from build123d import *

# Parameters (mm, degrees)
BOSS_EXTRUDE1_DEPTH           = 10
FILLET1_R                     = 5
CHAMFER1_SIZE                 = 1.5
CSK_FOR_M4_SFHCS1_D           = 4.8
CSK_FOR_M4_SFHCS1_CSINK_D     = 8.96
CSK_FOR_M4_SFHCS1_CSINK_ANGLE = 90
CSK_FOR_M4_SFHCS2_D           = 4.8
CSK_FOR_M4_SFHCS2_DEPTH       = 9.6
CSK_FOR_M4_SFHCS2_CSINK_D     = 8.96
CSK_FOR_M4_SFHCS2_CSINK_ANGLE = 90


with BuildPart() as part:
    # Sketch1 → Boss-Extrude1 (new body)
    with BuildSketch(Plane(origin=(0, 0, 0), x_dir=(1, 0, 0), z_dir=(0, 1, 0))):
        Polygon((-30, -17.5), (-30, -27.5), (30, -27.5), (30, -17.5), (20, -17.5), (20, 27.5), (10.4, 27.5), (10.4, 7.1), (-10.4, 7.1), (-10.4, 27.5), (-20, 27.5), (-20, -17.5), align=None)
    extrude(amount=BOSS_EXTRUDE1_DEPTH)

    # Fillet1
    fillet1_edges = [part.edges().sort_by_distance(p)[0] for p in [
        (-15.2, 0, -27.5),
        (15.2, 0, -27.5),
        (-15.2, 10, -27.5),
        (15.2, 10, -27.5),
        (0, 10, -7.1),
        (0, 0, -7.1),
    ]]
    fillet(fillet1_edges, radius=FILLET1_R - 0.0001)  # a hair under: the kernel refuses the full size

    # Chamfer1
    chamfer1_edges = [part.edges().sort_by_distance(p)[0] for p in [
        (30, 0, 22.5),
        (-30, 0, 22.5),
        (-30, 10, 22.5),
        (30, 10, 22.5),
    ]]
    chamfer(chamfer1_edges, length=CHAMFER1_SIZE)

    # CSK for M4 SFHCS1 (through all)
    with Locations(Plane(origin=(0, 0, 17.5), x_dir=(-1, 0, 0), z_dir=(0, 0, -1))):
        with Locations((-25, 5), (25, 5)):
            CounterSinkHole(CSK_FOR_M4_SFHCS1_D / 2, CSK_FOR_M4_SFHCS1_CSINK_D / 2, counter_sink_angle=CSK_FOR_M4_SFHCS1_CSINK_ANGLE)

    # CSK for M4 SFHCS2
    with Locations(Plane.ZY.offset(20)):
        with Locations((-22.5, 5)):
            csk_for_m4_sfhcs2 = CounterSinkHole(CSK_FOR_M4_SFHCS2_D / 2, CSK_FOR_M4_SFHCS2_CSINK_D / 2, depth=CSK_FOR_M4_SFHCS2_DEPTH, counter_sink_angle=CSK_FOR_M4_SFHCS2_CSINK_ANGLE)

    # Mirror1: CSK for M4 SFHCS2 across plane
    add(csk_for_m4_sfhcs2.mirror(Plane(origin=(0, 0, 0), x_dir=(0, 0, 1), z_dir=(1, 0, 0))), mode=Mode.SUBTRACT)


solid = part.part
Geometry check sheet. Reference: the model listing, model coordinates, mm. A direction names the side the tool comes from. Give positions to 0.01 mm unless a question says otherwise; leave off trailing zeros. Write each loop counter-clockwise with the first axis right and the second up, starting at its lowest first coordinate (ties: lowest second). Pieces come first, ordered by that corner, then holes. Notation, with made-up numbers: M 32.5,49 L 84.5,49 A22 ccw 84.5,55 Z; hole C -14,69 d5. An arc over 180 degrees is marked long. Answer as CSV lines item,"result". Start each with the question number.
Q1. Section check A-A, the plane x = 25. Record the cut outline in (y, z).
Q2. Section check B-B, the plane z = 22. Record the cut outline in (x, y), then the cut area to 3 significant figures.
Q3. Go/stop test with flat-tipped pins: pin 1 (5 mm diameter, centred on x = 25.5, y = 3, fed in from -Z); pin 2 (3 mm diameter, centred on x = -26, y = 6.5, fed in from -Z); pin 3 (5 mm diameter, centred on y = 1, z = 3.5, fed in from +X). Record where each tip stops, or that it passes through.
Q4. Tool access check on faces 1 (the face through (-20.5, 3.8, 17.5)), 2 (the face through (-0.15, 8.5, -5.67)), 3 (the face through (0, 0, 8)), 4 (the face through (23.959, 0.486, 17.5)). Record the directions out of +Z, -Z, +X, -X, +Y, -Y that give a thin tool (end or side, any length) a straight path to the whole face; none if there is none.
Q5. Material ranges on L1, parallel to X at y = 5, z = 24; L2, parallel to X at y = 9.75, z = -8.5; L3, parallel to Y at x = 16.5, z = -22.5, recorded low to high.
Q6. Release check for a two-part mould opening along Y. For faces 5 (the face through (-15.27, 8.5, -26.07)), 6 (the face through (14.11, 5.72, -24.79)), 7 (the face through (-20, 5, 0)) record: pulls with the +Y half, pulls with the -Y half, needs draft (parallel to the pull), parting line crosses it, or undercut.
Geometry says:
1,outline,"M 0,17.5 L 0.52,17.5 L 2.6,19.58 L 2.6,27.5 L 0,27.5 Z; M 7.4,19.58 L 9.48,17.5 L 10,17.5 L 10,27.5 L 7.4,27.5 Z"
2,outline,"M -30,1.5 L -28.5,0 L 28.5,0 L 30,1.5 L 30,8.5 L 28.5,10 L -28.5,10 L -30,8.5 Z; hole C -25,5 d4.8; hole C 25,5 d4.8"
2,area,"559 mm^2"
3,pin 1,"z = 17.5"
3,pin 2,"z = 18.68"
3,pin 3,"x = 20"
4,face 1,"-Z, -X, +Y, -Y"
4,face 2,"-Z, +Y"
4,face 3,"+Z, -Z, +X, -X, -Y"
4,face 4,"-Z, +X, +Y, -Y"
5,L1,"-30 to -27.4, -22.6 to 22.6, 27.4 to 30"
5,L2,"-20 to -10.4, 10.4 to 20"
5,L3,"0 to 2.6, 7.4 to 10"
6,face 5,"pulls with the +Y half"
6,face 6,"undercut"
6,face 7,"needs draft"
